from build123d import *

# Parameters (mm, degrees)
SKETCH1_W = 8.257122183
SKETCH1_H = 10
SKETCH1_R = 1.5


with BuildPart() as part:
    # Sketch1 → Revolve10 (revolve)
    with BuildSketch(Plane(origin=(0, 0, 0), x_dir=(1, 0, 0), z_dir=(0, 1, 0)), mode=Mode.PRIVATE) as revolve10_sk:
        Polygon((0, 48.49231552), (0, 0), (5, 0), (5, 15), (38.242877817, 15), (38.242877817, 25), (30, 25), (30, 48.49231552), (25, 48.49231552), (16.449496417, 25), (13.550503583, 25), (5, 48.49231552), align=None)
        with Locations((45.871438908, 20)):
            Rectangle(SKETCH1_W, SKETCH1_H)
        Polygon((38.242877817, 25), (38.242877817, 15), (39.242877817, 15), (40.742877817, 15), (41.742877817, 15), (41.742877817, 25), (40.75, 25), (40.742877817, 25), (39.25, 25), (39.242877817, 25), align=None)
        with Locations((40, 20.511791121)):
            Circle(SKETCH1_R, mode=Mode.SUBTRACT)
    revolve(revolve10_sk.sketch.rotate(Axis((0, 0, 0), (1, 0, 0)), 180), axis=Axis((0, 0, 0), (1, 0, 0)))


solid = part.part
Input: part model. Units: mm. Frame: model coordinates. A direction names the side the tool comes from. Give positions to 0.01 mm unless a question says otherwise; leave off trailing zeros. Write each loop counter-clockwise with the first axis right and the second up, starting at its lowest first coordinate (ties: lowest second). Pieces come first, ordered by that corner, then holes. Notation, with made-up numbers: (-3.75, -31.75) -> (27.25, -31.75) arc R24 cw to (27.25, -15.75) -> close; hole circle Ø8 at (79, 75). An arc over 180 degrees is marked (long way). Use one line per item in the form item = value. Start each with the question number.
1) Section query B-B on x = 15. Return the cut outline in (y, z).
2) Pin query (flat end, axial travel): pin 1 (8 mm diameter, centred on y = -17.5, z = -9.5, fed in from -X); pin 2 (1.5 mm diameter, centred on x = 42, z = 19.5, fed in from -Y); pin 3 (5 mm diameter, centred on x = 7, z = 15.5, fed in from -Y); pin 4 (12 mm diameter, centred on x = 45, z = -33, fed in from +Y). Return the tip coordinate at first contact, or that it passes through.
3) Draft query along X for faces 1 (the flat face through (50, 11, -11)), 2 (the flat face through (0, -1, -1)), 3 (the cylindrical face through (2.465, -2.132, -48.445)), 4 (the conical face through (13.016, -26.244, -3.446)). Return one class per face: pulls with the +X half, pulls with the -X half, needs draft (parallel to the pull), parting line crosses it, or undercut.
4) Section query D-D on x = 28. Return the cut outline in (y, z), then the cut area to 3 significant figures.
5) Set-up query: faces 5 (the cylindrical face through (27.465, -2.132, -48.445)), 6 (the flat face through (30, 21, -21)), 7 (the cylindrical face through (14.98, -7.509, 23.846)). Return all of +Z, -Z, +X, -X, +Y, -Y with unobstructed straight access to the full face (end or side cutting, diameter ignored); none if empty.
6) Ray query, probe 1 along Y at (x, z) = (28, 0); probe 2 along Y at (x, z) = (33, 0); probe 3 along X at (y, z) = (-27.5, 1). Return the intervals inside material, ascending. Write a range as from..to.
7) Section query A-A on y = 0. Return the cut outline in (x, z), then the cut area to 3 significant figures.
Outcome:
q1.outline = circle Ø50 at (0, 0); hole circle Ø30 at (0, 0)
q2.pin_1 = 0
q2.pin_2 = -16.54
q2.pin_3 = -46.43
q2.pin_4 = through
q3.face_1 = pulls with the +X half
q3.face_2 = pulls with the -X half
q3.face_3 = needs draft
q3.face_4 = undercut
q4.outline = circle Ø96.98 at (0, 0); hole circle Ø30 at (0, 0)
q4.area = 6,680 mm^2
q5.face_5 = +X, -X
q5.face_6 = +X
q5.face_7 = none
q6.probe_1 = -48.49..-15, 15..48.49
q6.probe_2 = -25..-15, 15..25
q6.probe_3 = 0..12.63, 17.37..30
q7.outline = (0, -48.49) -> (5, -48.49) -> (13.55, -25) -> (16.45, -25) -> (25, -48.49) -> (30, -48.49) -> (30, -25) -> (50, -25) -> (50, -15) -> (5, -15) -> (5, 15) -> (50, 15) -> (50, 25) -> (30, 25) -> (30, 48.49) -> (25, 48.49) -> (16.45, 25) -> (13.55, 25) -> (5, 48.49) -> (0, 48.49) -> close; hole circle Ø3 at (40, -20.51); hole circle Ø3 at (40, 20.51)
q7.area = 2,010 mm^2
